For this review, take the finished solid that the model builds, in its own axes (mm). A direction names the side the tool comes from. Coordinates: 2 decimals unless noted, no trailing zeros. Loops run counter-clockwise (first coordinate to the right, second up) from the corner with the lowest first, then second, coordinate; pieces in that order, holes last. Notation, with made-up numbers: (-13, -14) -> (22, -14) arc R12 ccw to (22, -7) -> close; hole circle Ø11 at (-26.5, 20.5). An arc over 180 degrees is marked (long way). Answer in a Markdown table with one row per item.
from build123d import *

# Parameters (mm, degrees)
SKETCH1_R           = 1.65
BOSS_EXTRUDE1_DEPTH = 10
CUT_EXTRUDE1_START  = -2
SKETCH2_R           = 2.5
CUT_EXTRUDE1_DEPTH  = 10
SKETCH3_W           = 1
SKETCH3_H           = 8
CUT_EXTRUDE2_DEPTH  = 0.6
FILLET1_R           = 0.5


with BuildPart() as part:
    # Sketch1 → Boss-Extrude1 (new body)
    with BuildSketch(Plane(origin=(0, 0, 0), x_dir=(1, 0, 0), z_dir=(0, 1, 0))):
        with BuildLine():
            Line((4.25, 21.3), (4.25, -11.755317946))
            ThreePointArc((4.25, -11.755317946), (2.157374061, -12.312422067), (0, -12.5))
            Line((0, -12.5), (-0.6, -2.939387691))
            ThreePointArc((-0.6, -2.939387691), (-2.323790008, -1.897366596), (-3, 0))
            Line((-3, 0), (-3, 5))
            Line((-3, 5), (-0.6, 5.5))
            Line((-0.6, 5.5), (-0.6, 15.126776243))
            Line((-0.6, 15.126776243), (0, 15.020980054))
            ThreePointArc((0, 15.020980054), (1.731070844, 16.737548219), (-0.45, 17.826649916))
            Line((-0.45, 17.826649916), (-0.6, 17.826649916))
            Line((-0.6, 17.826649916), (-0.6, 20.3))
            Line((-0.6, 20.3), (0.4, 21.3))
            Line((0.4, 21.3), (4.25, 21.3))
        make_face()
        with Locations(Location((0, 0, 0), (0, 0, 270))):
            Circle(SKETCH1_R, mode=Mode.SUBTRACT)
    extrude(amount=BOSS_EXTRUDE1_DEPTH)

    # Sketch2 → Cut-Extrude1 (cut)
    with BuildSketch(Plane(origin=(4.25, 0, 0), x_dir=(0, 0, -1), z_dir=(1, 0, 0)).offset(CUT_EXTRUDE1_START)):
        with Locations((-7, 5)):
            Circle(SKETCH2_R)
    extrude(amount=-CUT_EXTRUDE1_DEPTH, mode=Mode.SUBTRACT)

    # Sketch3 → Cut-Extrude2 (cut)
    with BuildSketch(Plane(origin=(4.25, 0, 0), x_dir=(0, 0, -1), z_dir=(1, 0, 0))):
        with Locations((-10.255317946, 5)):
            Rectangle(SKETCH3_W, SKETCH3_H)
        with Locations((-8.255317946, 5)):
            Rectangle(SKETCH3_W, SKETCH3_H)
        with Locations((-6.255317946, 5)):
            Rectangle(SKETCH3_W, SKETCH3_H)
        with Locations((-4.255317946, 5)):
            Rectangle(SKETCH3_W, SKETCH3_H)
    extrude(amount=-CUT_EXTRUDE2_DEPTH, mode=Mode.SUBTRACT)

    # Fillet1
    fillet1_edges = [part.edges().sort_by_distance(p)[0] for p in [
        (3.65, 5, 10.755317946),
        (3.65, 9, 10.255317946),
        (3.65, 5, 9.755317946),
        (3.65, 1, 10.255317946),
        (3.65, 5, 8.755317946),
        (3.65, 9, 8.255317946),
        (3.65, 5, 7.755317946),
        (3.65, 1, 8.255317946),
        (3.65, 5, 6.755317946),
        (3.65, 9, 6.255317946),
        (3.65, 5, 5.755317946),
        (3.65, 1, 6.255317946),
        (3.65, 5, 4.755317946),
        (3.65, 9, 4.255317946),
        (3.65, 5, 3.755317946),
        (3.65, 1, 4.255317946),
    ]]
    fillet(fillet1_edges, radius=FILLET1_R - 0.0001)  # a hair under: the kernel refuses the full size


solid = part.part
Item 1: Take a section at B-B, the plane z = -16.5. State the section outline as (x, y) points, and give its area (3 significant figures).
Worked answers:
| item | result |
|---|---|
| outline | (1.75, 0) -> (4.25, 0) -> (4.25, 10) -> (1.75, 10) -> close |
| area | 25.0 mm² |
Item 2: For faces 4 (the flat face through (-0.6, 5, -19)), 5 (the cylindrical face through (0.893, 5.751, 4.615)), 6 (the cylindrical face through (-2.305, 4.93, 1.92)), list the 3-axis set-ups (+Z, -Z, +X, -X, +Y, -Y) from which the entire face can be reached by the end or side of a thin tool; tool diameter is ignored.
Worked answers:
| item | result |
|---|---|
| face 4 | -Z, -X, +Y, -Y |
| face 5 | -X |
| face 6 | +Z, -X, +Y, -Y |
Item 3: For L1, parallel to Y at x = 1.6, z = 7; L2, parallel to Z at x = 0.5, y = 1; L3, parallel to Z at x = 0.25, y = 4, list the stretches that pass through material, from the lowest coordinate up.
Worked answers:
| item | result |
|---|---|
| L1 | 0 to 2.5, 7.5 to 10 |
| L2 | -21.3 to -17.98, -15.02 to -1.57, 1.57 to 12.49 |
| L3 | -21.15 to -18, -15 to -1.63, 1.63 to 4.71, 9.29 to 12.5 |
Item 4: Insertion check: pin 1 (1 mm diameter, centred on y = 7, z = 2.5, fed in from -X); pin 2 (1.2 mm diameter, centred on y = 3.5, z = -18.5, fed in from -X). Each pin has a flat end and moves straight along its axis. Give the tip position at first contact, or say it passes through.
Worked answers:
| item | result |
|---|---|
| pin 1 | x = -2.24 |
| pin 2 | x = -0.6 |
Item 5: The part is to be moulded in two halves that separate along X. For faces 1 (the cylindrical face through (-1, 4.93, -1.31)), 2 (the flat face through (4.25, 5, -5)), 3 (the flat face through (1, 0, -5)), say which applies: +X half, -X half, draft (parallel to the pull), parting line (faces both ways), or undercut.
Worked answers:
| item | result |
|---|---|
| face 1 | undercut |
| face 2 | +X half |
| face 3 | draft |
Item 6: Take a section at A-A, the plane z = -9. State the section outline as (x, y) points.
Worked answers:
| item | result |
|---|---|
| outline | (-0.6, 0) -> (4.25, 0) -> (4.25, 10) -> (-0.6, 10) -> close |
